Autodesk Inventor part; units mm, degrees
ref_plane "YZ Plane" through (0, 0, 0) normal (1, 0, 0) x (0, 1, 0)
ref_plane "XZ Plane" through (0, 0, 0) normal (0, 1, 0) x (-1, 0, 0)
ref_plane "XY Plane" through (0, 0, 0) normal (0, 0, 1) x (1, 0, 0)
sketch "Sketch1" plane through (0, 0, 0) normal (0, 1, 0) x (-1, 0, 0)
  line L0 (-44.45, -19.05) -> (44.45, -19.05)
  line L1 (44.45, -19.05) -> (44.45, 19.05)
  line L2 (44.45, 19.05) -> (-44.45, 19.05)
  line L3 (-44.45, 19.05) -> (-44.45, -19.05)
  line L4 (-44.45, -19.05) -> (44.45, 19.05) construction
  line L5 (44.45, -19.05) -> (-44.45, 19.05) construction
  circle A0 centre (22.225, 0) radius 3.9688
  circle A1 centre (-22.225, 0) radius 3.9688
  circle A2 centre (22.225, 0) radius 12.7
  circle A3 centre (-22.225, 0) radius 12.7
  point P0 (0, 0)
  point P1 (0, 0)
  point P2 (0, 0)
  dimension "d3" = 38.1
  dimension "d4" = 88.9
  dimension "d20" = 7.9375
  dimension "d21" = 25.4
  dimension "d22" = 22.225
  dimension "d23" = 22.225
extrude "Extrusion5" add sketch "Sketch1" along normal blind 50.8 contours L3 L2 L1 L0 | A2 | A3
sketch "Sketch10" plane through (0, 50.8, 0) normal (0, 1, 0) x (1, 0, 0)
  circle A0 centre (22.225, 0) radius 3.9687
  circle A1 centre (-22.225, 0) radius 3.9687
  line L0 (44.45, 19.05) -> (-44.45, 19.05)
  line L1 (-44.45, 19.05) -> (-44.45, -19.05)
  line L2 (-44.45, -19.05) -> (44.45, -19.05)
  line L3 (44.45, -19.05) -> (44.45, 19.05)
  circle A2 centre (-22.225, 0) radius 4.826
  circle A3 centre (-22.225, 0) radius 9.525
  point P0 (0, 0)
  dimension "d38" = 9.652
  dimension "d41" = 19.05
extrude "Extrusion8" cut sketch "Sketch10" against normal blind 38.1 contours A2
extrude "Extrusion9" cut sketch "Sketch10" against normal blind 25.4 contours A3
sketch "Sketch12" plane through (0, 50.8, 0) normal (0, 1, 0) x (1, 0, 0)
  circle A0 centre (-22.225, 0) radius 9.525
  circle A1 centre (22.225, 0) radius 3.9687
  line L0 (44.45, 19.05) -> (-44.45, 19.05)
  line L1 (-44.45, 19.05) -> (-44.45, -19.05)
  line L2 (-44.45, -19.05) -> (44.45, -19.05)
  line L3 (44.45, -19.05) -> (44.45, 19.05)
  circle A2 centre (-22.225, 0) radius 3.9687
  line L4 (-22.225, 0) -> (22.225, 0) construction
  line L5 (-22.225, -9.525) -> (22.225, -9.525)
  line L6 (22.225, 9.525) -> (-22.225, 9.525)
  arc A3 (-22.225, 9.525) -> (-22.225, -9.525) centre (-22.225, 0) ccw
  arc A4 (22.225, -9.525) -> (22.225, 9.525) centre (22.225, 0) ccw
  point P0 (0, 0)
  point P1 (0, 0)
extrude "Extrusion10" cut sketch "Sketch12" against normal up to surface (25.4 mm away) contours A0 | A0 L6 A4 L5
properties part number "AirPressureAndValvePart2"
Could you check a few things on this model? Use its own coordinates, in mm. A direction names the side the tool comes from. Coordinates: 2 decimals unless noted, no trailing zeros. Write each loop counter-clockwise with the first axis right and the second up, starting at its lowest first coordinate (ties: lowest second). Pieces come first, ordered by that corner, then holes. Notation, with made-up numbers: (-24, 62.5) - (27, 62.5) arc R29 ccw to (27, 101.5) - close; hole circle Ø11 at (85.25, 45). An arc over 180 degrees is marked (long way). Write item = value, one per line.
1) Suppose I cut it at B-B on z = 0. Please give me the cut outline in (x, y).
Result set:
outline = (-44.45, 0) - (-26.19, 0) - (-26.19, 12.7) - (-27.05, 12.7) - (-27.05, 25.4) - (-31.75, 25.4) - (-31.75, 50.8) - (-44.45, 50.8) - close; (-18.26, 0) - (18.26, 0) - (18.26, 25.4) - (-17.4, 25.4) - (-17.4, 12.7) - (-18.26, 12.7) - close; (26.19, 0) - (44.45, 0) - (44.45, 50.8) - (31.75, 50.8) - (31.75, 25.4) - (26.19, 25.4) - close
2) We'd pull the mould along X, two halves only. Please class faces 1 (the flat face through (-1, 25, 19.05)), 2 (the flat face through (0, 25.4, 0)), 3 (the flat face through (44.45, 25, 0)): +X half, -X half, draft (parallel to the pull), parting line (faces both ways), or undercut.
Result set:
face_1 = draft
face_2 = undercut
face_3 = +X half
3) Suppose I cut it at C-C on x = -5. Please give me the cut outline in (y, z) (3 decimals).
Result set:
outline = (0, -19.05) - (50.8, -19.05) - (50.8, -9.525) - (25.4, -9.525) - (25.4, 9.525) - (50.8, 9.525) - (50.8, 19.05) - (0, 19.05) - close
4) For faces 4 (the cylindrical face through (-25.9, 6.3, 1.5)), 5 (the flat face through (0, 38, -9.525)), which set-ups out of +Z, -Z, +X, -X, +Y, -Y let a thin tool reach every point of the face, with its end or its side?
Result set:
face_4 = +Y, -Y
face_5 = +Y
5) Suppose I cut it at D-D on z = 6. Please give me the cut outline in (x, y), plus the area to 3 significant figures.
Result set:
outline = (-44.45, 0) - (44.45, 0) - (44.45, 50.8) - (29.62, 50.8) - (29.62, 25.4) - (-29.62, 25.4) - (-29.62, 50.8) - (-44.45, 50.8) - close
area = 3,010 mm2
6) Will these pins go through, and if not, where does the flat tip stop? pin 1 Ø1 at (x, z) = (-13, -1.5) entering from -Y; pin 2 Ø10.5 at (x, z) = (22.225, 0) entering from +Y; pin 3 Ø5 at (x, z) = (-22.225, 0) entering from -Y.
Result set:
pin_1 = 0
pin_2 = 25.4
pin_3 = through
7) Please list where these lines run through material, in increasing order: line 1 (X direction, y = 10.5, z = 0); line 2 (X direction, y = 19.25, z = 0); line 3 (Z direction, x = 0, y = 48) (3 decimals). Write a range as [from, to].
Result set:
line_1 = [-44.45, -26.19], [-18.26, 18.26], [26.19, 44.45]
line_2 = [-44.45, -27.05], [-17.4, 18.26], [26.19, 44.45]
line_3 = [-19.05, -9.525], [9.525, 19.05]
8) Suppose I cut it at A-A on y = 8. Please give me the cut outline in (x, z) (3 decimals), plus the area to 3 significant figures.
Result set:
outline = (-44.45, -19.05) - (44.45, -19.05) - (44.45, 19.05) - (-44.45, 19.05) - close; hole circle Ø7.938 at (-22.225, 0); hole circle Ø7.938 at (22.225, 0)
area = 3,290 mm2
